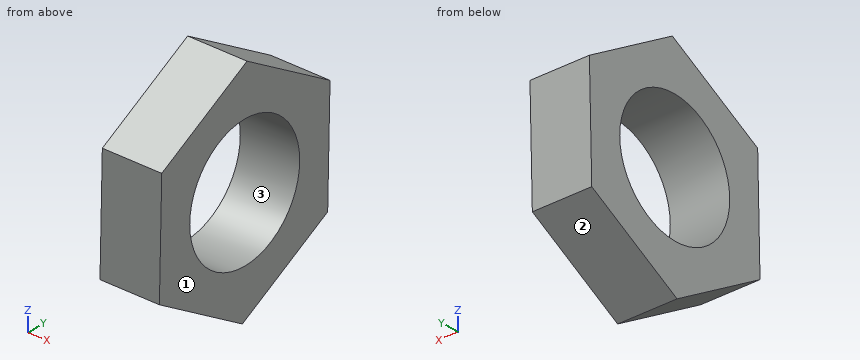
```python
from build123d import *

# Parameters (mm, degrees)
SKETCH1_R           = 10.322814
BOSS_EXTRUDE1_DEPTH = 9.490202


with BuildPart() as part:
    # Sketch1 → Boss-Extrude1 (new body)
    with BuildSketch(Plane(origin=(0, 0, 0), x_dir=(0, 0, -1), z_dir=(1, 0, 0))):
        Polygon((345.91117, 35.58921), (354.648291413, 19.572151802), (372.888031413, 19.130191802), (382.39065, 34.70529), (373.653528587, 50.722348198), (355.413788587, 51.164308198), align=None)
        with Locations((364.15091, 35.14725)):
            Circle(SKETCH1_R, mode=Mode.SUBTRACT)
    extrude(amount=-BOSS_EXTRUDE1_DEPTH)


solid = part.part
```
Verification items for the finished model (mm, model axes). Face numbers are marked on the shaded views. Coordinates: 2 decimals unless noted, no trailing zeros. Write each loop counter-clockwise with the first axis right and the second up, starting at its lowest first coordinate (ties: lowest second). Pieces come first, ordered by that corner, then holes. Notation, with made-up numbers: (-19, -14) - (4, -14) arc R14 ccw to (4, 5) - close; hole circle Ø8 at (73, 36). An arc over 180 degrees is marked (long way). Write item = value, one per line.
Q1. Mould release check, pull along Z, two halves, no side actions. Record for the marked faces 1, 2 and 3: released by +Z, released by -Z, zero draft, split by the parting line, or undercut.
Answer:
face_1 = zero draft
face_2 = released by -Z
face_3 = undercut
Q2. Cross-section at A-A (z = -368). Enter the section's corners in (x, y), plus the area to 3 significant figures.
Answer:
outline = (-9.49, 19.25) - (0, 19.25) - (0, 25.57) - (-9.49, 25.57) - close; (-9.49, 44.73) - (0, 44.73) - (0, 50.86) - (-9.49, 50.86) - close
area = 118 mm²
Q3. Cross-section at D-D (z = -379). Enter the section's corners in (x, y).
Answer:
outline = (-9.49, 29.15) - (0, 29.15) - (0, 40.92) - (-9.49, 40.92) - close
Q4. Cross-section at C-C (x = -7.75). Enter the section's corners in (y, z), plus the area to 3 significant figures.
Answer:
outline = (19.13, -372.89) - (34.71, -382.39) - (50.72, -373.65) - (51.16, -355.41) - (35.59, -345.91) - (19.57, -354.65) - close; hole circle Ø20.65 at (35.15, -364.15)
area = 530 mm²
Q5. Material ranges on L1, parallel to Y at x = -2, z = -360; L2, parallel to Z at x = -1.5, y = 40; L3, parallel to Y at x = -7.5, z = -369, recorded low to high. Write a range as from..to.
Answer:
L1 = 19.44..25.7, 44.6..51.05
L2 = -379.5..-373.26, -355.04..-348.6
L3 = 19.22..26.03, 44.26..50.84
Q6. Cross-section at B-B (y = 29). Enter the section's corners in (x, z), plus the area to 3 significant figures.
Answer:
outline = (-9.49, -378.91) - (0, -378.91) - (0, -372.44) - (-9.49, -372.44) - close; (-9.49, -355.86) - (0, -355.86) - (0, -349.51) - (-9.49, -349.51) - close
area = 122 mm²
Q7. Go/stop test with flat-tipped pins: pin 1 Ø4 at (x, z) = (-5.5, -351) entering from +Y; pin 2 Ø5 at (x, z) = (-7, -362.5) entering from +Y. Record where each tip stops, or that it passes through.
Answer:
pin_1 = 47.21
pin_2 = 51.05
